```python
from build123d import *

# Parameters (mm, degrees)
BOSS_EXTRUDE1_DEPTH = 16
CHAMFER1_SIZE       = 12
SKETCH2_R           = 1.6
CUT_EXTRUDE1_DEPTH  = 20
SKETCH2_4_R         = 3
SKETCH2_4_R_2       = 1.6
CUT_EXTRUDE2_DEPTH  = 16
CHAMFER2_SIZE       = 2


with BuildPart() as part:
    # Sketch1 → Boss-Extrude1 (new body)
    with BuildSketch(Plane(origin=(0, 0, 0), x_dir=(1, 0, 0), z_dir=(0, 1, 0))):
        with BuildLine():
            Line((-34.485549133, -2.028901734), (-44.485549133, -2.028901734))
            Line((-44.485549133, -2.028901734), (-44.485549133, 17.971098266))
            Line((-44.485549133, 17.971098266), (1.514450867, 17.971098266))
            Line((1.514450867, 17.971098266), (1.514450867, -2.028901734))
            Line((1.514450867, -2.028901734), (-8.485549133, -2.028901734))
            ThreePointArc((-8.485549133, -2.028901734), (-21.485549133, 10.971098266), (-34.485549133, -2.028901734))
        make_face()
    extrude(amount=BOSS_EXTRUDE1_DEPTH)

    # Chamfer1
    chamfer1_edges = [part.edges().sort_by_distance(p)[0] for p in [
        (-44.485549133, 8, -17.971098266),
        (1.514450867, 8, -17.971098266),
    ]]
    chamfer(chamfer1_edges, length=CHAMFER1_SIZE)

    # Sketch2 → Cut-Extrude1 (cut)
    with BuildSketch(Plane(origin=(0, 0, -17.971098266), x_dir=(-1, 0, 0), z_dir=(0, 0, -1))):
        with Locations((39.485549133, 8)):
            Circle(SKETCH2_R)
        with Locations((3.485549133, 8)):
            Circle(SKETCH2_R)
    extrude(amount=-CUT_EXTRUDE1_DEPTH, mode=Mode.SUBTRACT)

    # Sketch2<4> → Cut-Extrude2 (cut)
    # profile 1 of 2: a face of its own
    with BuildSketch(Plane(origin=(0, 0, -17.971098266), x_dir=(-1, 0, 0), z_dir=(0, 0, -1))):
        with Locations((39.485549133, 8)):
            Circle(SKETCH2_4_R)
        with Locations((39.485549133, 8)):
            Circle(SKETCH2_4_R_2, mode=Mode.SUBTRACT)
    # profile 2 of 2: a face of its own
    with BuildSketch(Plane(origin=(0, 0, -17.971098266), x_dir=(-1, 0, 0), z_dir=(0, 0, -1))):
        with Locations((3.485549133, 8)):
            Circle(SKETCH2_4_R)
        with Locations((3.485549133, 8)):
            Circle(SKETCH2_4_R_2, mode=Mode.SUBTRACT)
    extrude(amount=-CUT_EXTRUDE2_DEPTH, mode=Mode.SUBTRACT)

    # Chamfer2
    chamfer2_edges = [part.edges().sort_by_distance(p)[0] for p in [
        (1.514450867, 16, -1.971098266),
        (-21.485549133, 0, -17.971098266),
        (-21.485549133, 16, -17.971098266),
        (-44.485549133, 0, -1.971098266),
        (-38.485549133, 0, -11.971098266),
        (-4.485549133, 0, -11.971098266),
        (-44.485549133, 16, -1.971098266),
        (-38.485549133, 16, -11.971098266),
        (-4.485549133, 16, -11.971098266),
        (1.514450867, 0, -1.971098266),
    ]]
    chamfer(chamfer2_edges, length=CHAMFER2_SIZE)


solid = part.part
```
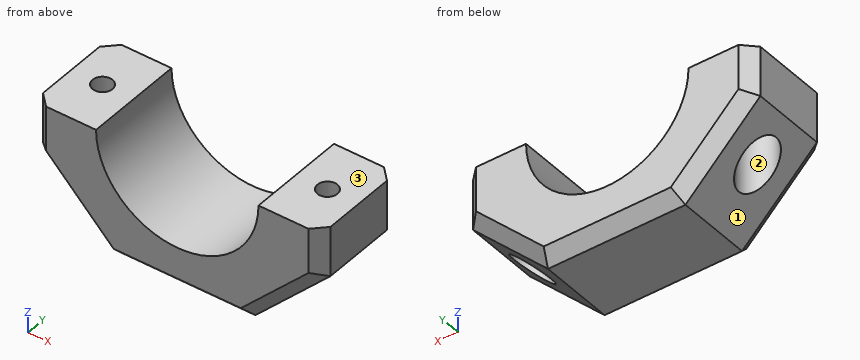
Here's how the part is built. I have some questions about the finished solid (model axes, mm). Face numbers are marked on the shaded views. Coordinates: 2 decimals unless noted, no trailing zeros. Write each loop counter-clockwise with the first axis right and the second up, starting at its lowest first coordinate (ties: lowest second). Pieces come first, ordered by that corner, then holes. Notation, with made-up numbers: (11, 55.5) - (28, 55.5) arc R37 cw to (28, 93.5) - close; hole circle Ø6 at (28, 16). An arc over 180 degrees is marked (long way). One line per item, written item: value.
1) Suppose I cut it at A-A on y = 7.25. Write out the boundary of the cut face in (x, z).
Model answer:
outline: (-44.49, -5.97) - (-42.39, -8.07) - (-42.39, -1.97) - (-40.9, -1.97) - (-40.9, 2.03) - (-44.49, 2.03) - close; (-38.07, -1.97) - (-36.58, -1.97) - (-36.58, -13.88) - (-32.49, -17.97) - (-10.49, -17.97) - (-6.39, -13.88) - (-6.39, -1.97) - (-4.9, -1.97) - (-4.9, 2.03) - (-8.49, 2.03) arc R13 cw to (-34.49, 2.03) - (-38.07, 2.03) - close; (-2.07, -1.97) - (-0.58, -1.97) - (-0.58, -8.07) - (1.51, -5.97) - (1.51, 2.03) - (-2.07, 2.03) - close
2) Suppose I cut it at D-D on x = -30. Write out the boundary of the cut face in (y, z).
Model answer:
outline: (0, -15.97) - (2, -17.97) - (14, -17.97) - (16, -15.97) - (16, -7.79) - (0, -7.79) - close
3) Suppose I cut it at C-C on x = -18. Write out the boundary of the cut face in (y, z), and give its area (3 significant figures).
Model answer:
outline: (0, -15.97) - (2, -17.97) - (14, -17.97) - (16, -15.97) - (16, -10.5) - (0, -10.5) - close
area: 116 mm²
4) Suppose I cut it at B-B on x = -39. Write out the boundary of the cut face in (y, z), and give its area (3 significant figures).
Model answer:
outline: (0, -8.63) - (2, -11.46) - (5.04, -11.46) - (5.04, -1.97) - (6.48, -1.97) - (6.48, 2.03) - (0, 2.03) - close; (9.52, -1.97) - (10.96, -1.97) - (10.96, -11.46) - (14, -11.46) - (16, -8.63) - (16, 2.03) - (9.52, 2.03) - close
area: 142 mm²
5) I'm going to push flat-ended pins straight in: P1, Ø3, axis at x = -7.5, z = -12.5, coming from the +Y side; P2, Ø5.5, axis at x = -39.49, y = 8, coming from the -Z side; P3, Ø4, axis at y = 6.5, z = -16, coming from the -X side; P4, Ø5, axis at y = 7.5, z = -15, coming from the -X side. Where does each tip first touch, or does it pass through?
Model answer:
P1: stops at y = 16
P2: stops at z = -1.97
P3: stops at x = -36.46
P4: stops at x = -37.36
6) I need wall thicknesses on line 1 along X through (y, z) = (8, -7); line 2 along Y through (x, z) = (-3.5, -3.75); line 3 along X through (y, z) = (8.75, -5). Which ranges of each line are inside material? Lowest first, please.
Model answer:
line 1: x = -43.46 to -42.49, -36.49 to -30.84, -12.13 to -6.49, -0.49 to 0.49
line 2: y = 0 to 5, 11 to 16
line 3: x = -44.49 to -42.39, -36.58 to -32.42, -10.55 to -6.39, -0.58 to 1.51
7) We'd pull the mould along X, two halves only. Please class the marked faces 1, 2 and 3: pulls with the +X half, pulls with the -X half, needs draft (parallel to the pull), parting line crosses it, or undercut.
Model answer:
face 1: pulls with the -X half
face 2: undercut
face 3: needs draft
